Autodesk Inventor part; units mm, degrees
ref_plane "YZ Plane" through (0, 0, 0) normal (1, 0, 0) x (0, 1, 0)
ref_plane "XZ Plane" through (0, 0, 0) normal (0, 1, 0) x (-1, 0, 0)
ref_plane "XY Plane" through (0, 0, 0) normal (0, 0, 1) x (1, 0, 0)
sketch "Sketch1" plane through (0, 0, 0) normal (1, 0, 0) x (0, 1, 0)
  line L0 (0, 0) -> (0, -540)
  line L1 (0, 0) -> (34, 0)
  line L2 (34, 0) -> (34, -340)
  line L3 (34, -340) -> (146, -340)
  line L4 (0, -540) -> (20, -540)
  line L5 (20, -540) -> (146, -340)
  dimension "d0" = 68
  dimension "d1" = 112
  dimension "d2" = 20
  dimension "d3" = 540
  dimension "d4" = 340
revolve "Revolution1" add sketch "Sketch1" angle 360 about axis through (0, 0, 0) along (0, 0, -1)
fillet "Fillet1" radius 20 1 edges at (0, -20, -540)
fillet "Fillet2" radius 1 1 edges at (0, -146, -340)
properties part number "ConoEntrata" material "Steel, Alloy"
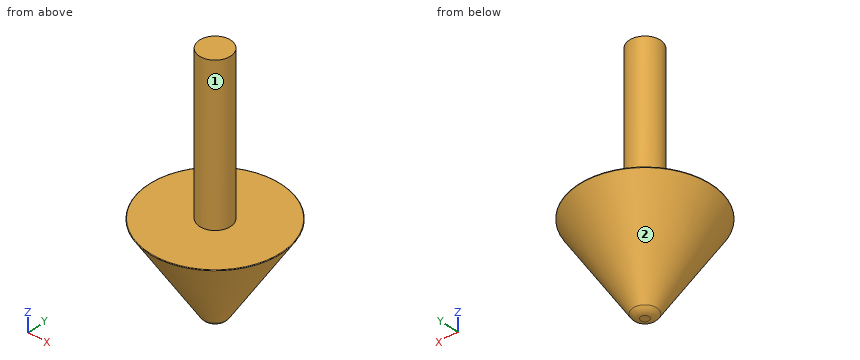
Build history of the part. All positions in model axes, mm. Face numbers are marked on the shaded views. A direction names the side the tool comes from. Give positions to 0.01 mm unless a question says otherwise; leave off trailing zeros. Loops run counter-clockwise (first coordinate to the right, second up) from the corner with the lowest first, then second, coordinate; pieces in that order, holes last.
1) Band-saw the part on A-A on z = -501. List the corners of the cut face in (x, y), then the cut area to 3 significant figures.
Values follow:
outline: circle Ø89.14 at (0, 0)
area: 6,240 mm2
2) Probe line 1 along Y through (x, z) = (1, -258); line 2 along Z through (x, y) = (111.5, 76.5); line 3 along Z through (x, y) = (-92.5, -82). List the from-to ranges inside material, lowest first.
Values follow:
line 1: y = -33.99 to 33.99
line 2: z = -357.11 to -340
line 3: z = -375.53 to -340
3) Band-saw the part on B-B on z = -229. List the corners of the cut face in (x, y).
Values follow:
outline: circle Ø68 at (0, 0)
4) 3-axis set-ups, long thin cutter, end or side, ignore diameter. For the marked faces 1 and 2: which of +Z, -Z, +X, -X, +Y, -Y reach the whole face in a straight line?
Values follow:
face 1: +Z
face 2: -Z
5) Drop flat-ended pins along their axis: P1, Ø8, axis at x = -62.5, z = -401.5, coming from the -Y side; P2, Ø4, axis at x = 86.5, y = 89.5, coming from the -Z side; P3, Ø3, axis at x = -107.5, y = 42.5, coming from the +Z side. Give the stop position or say it passes through.
Values follow:
P1: stops at y = -91.27
P2: stops at z = -377.35
P3: stops at z = -340
